Source: CAD feature listing. Evaluate the final solid. Frame: model axes, mm. Face numbers are marked on the shaded views. A direction names the side the tool comes from. Round coordinates to 2 decimals unless told otherwise and drop trailing zeros. Order: outer loops, then holes, each group sorted by start corner. A loop starts at its lowest first (then second) coordinate and runs counter-clockwise, first axis right, second up. Notation, with made-up numbers: (56, 32.5) - (97, 32.5) arc R23 cw to (97, 54.5) - close; hole circle Ø9 at (36, 33). An arc over 180 degrees is marked (long way). Return JSON: item names as keys, results as strings. Group by question number.
1) Mould query, pull axis X, two halves, no side actions, for the marked faces 4, 5 and 6. Classes: pulls with the +X half, pulls with the -X half, needs draft (parallel to the pull), parting line crosses it, or undercut.
2) Section D-D, the plane y = -17.5. Return loops of the section in (x, z).
3) Section B-B, the plane y = -5.5. Return loops of the section in (x, z).
4) Ray query, line 1 (Y direction, x = 7.25, z = 7); line 2 (X direction, y = 0, z = 9.75); line 3 (Z direction, x = -16, y = -18). Return the intervals inside material, ascending. Write a range as from..to.
5) Access query for the marked faces 1, 2 and 3. Directions: +Z, -Z, +X, -X, +Y, -Y. A direction counts if a zero-diameter tool reaches every point of the face in a straight line with its end or side. Return the directions, or none.
6) Section A-A, the plane x = -16. Return loops of the section in (y, z), plus the area to 3 significant figures.
7) Contact query for flat-ended pins moving along their axis: P1, Ø5, axis at x = 16, z = 7, coming from the +Y side; P2, Ø2.5, axis at y = 11.5, z = 5.5, coming from the -X side; P3, Ø2.5, axis at y = 9.5, z = 7.5, coming from the +X side; P4, Ø3.5, axis at x = 14.5, z = 8, coming from the +Y side. Output: stop coordinate, or through.
8) Section C-C, the plane z = 2. Return loops of the section in (x, y).
```python
from build123d import *

# Parameters (mm, degrees)
BOSS_EXTRUDE1_DEPTH         = 14
TAP_DRILL_FOR_M4X0_7_TAP2_D = 3.3
F_12_0_12_DIAMETER_HOLE1_D  = 12
TAP_DRILL_FOR_M5X0_8_TAP1_D = 5.5


with BuildPart() as part:
    # Sketch2 → Boss-Extrude1 (new body)
    with BuildSketch(Plane.XY):
        Polygon((-1, 0), (-1, 14.5), (-9, 14.5), (-9, -17), (-21, -17), (-21, -23), (0, -23), (0, 0), align=None)
    boss_extrude1 = extrude(amount=BOSS_EXTRUDE1_DEPTH)

    # Mirror1: Boss-Extrude1 across plane
    add(boss_extrude1.mirror(Plane(origin=(0, -23, 14), x_dir=(0, 0, 1), z_dir=(-1, 0, 0))))

    # Tap Drill for M4x0.7 Tap2 (through all)
    with Locations(Plane.ZY.offset(9)):
        with Locations((7, 10)):
            Hole(TAP_DRILL_FOR_M4X0_7_TAP2_D / 2)

    # Ø12.0 (12) Diameter Hole1 (through all)
    with Locations(Plane(origin=(0, 0, 0), x_dir=(1, 0, 0), z_dir=(0, 0, -1))):
        with Locations((0, 0)):
            Hole(F_12_0_12_DIAMETER_HOLE1_D / 2)

    # Tap Drill for M5x0.8 Tap1 (through all)
    with Locations(Plane(origin=(0, -23, 0), x_dir=(-1, 0, 0), z_dir=(0, -1, 0))):
        with Locations((-16, -7), (16, -7)):
            Hole(TAP_DRILL_FOR_M5X0_8_TAP1_D / 2)


solid = part.part
```
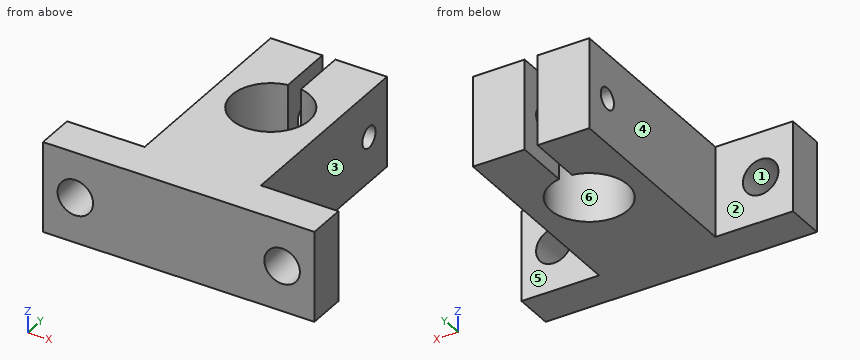
Geometry check:
{
 "1": {"face 4": "pulls with the -X half", "face 5": "needs draft", "face 6": "undercut"},
 "2": {"outline": "(-21, 0) - (21, 0) - (21, 14) - (-21, 14) - close; hole circle Ø5.5 at (-16, 7); hole circle Ø5.5 at (16, 7)"},
 "3": {"outline": "(-9, 0) - (-2.4, 0) - (-2.4, 14) - (-9, 14) - close; (2.4, 0) - (9, 0) - (9, 14) - (2.4, 14) - close"},
 "4": {"line 1": "-23..8.35, 11.65..14.5", "line 2": "-9..-6, 6..9", "line 3": "0..4.25, 9.75..14"},
 "5": {"face 1": "+Y, -Y", "face 2": "+Z, -Z, -X, +Y", "face 3": "+Z, -Z, +X, +Y"},
 "6": {"outline": "(-23, 0) - (-17, 0) - (-17, 4.25) - (-23, 4.25) - close; (-23, 9.75) - (-17, 9.75) - (-17, 14) - (-23, 14) - close", "area": "51.0 mm2"},
 "7": {"P1": "through", "P2": "x = -9", "P3": "x = 9", "P4": "y = -17"},
 "8": {"outline": "(-21, -23) - (21, -23) - (21, -17) - (9, -17) - (9, 14.5) - (1, 14.5) - (1, 5.92) arc R6 cw (long way) to (-1, 5.92) - (-1, 14.5) - (-9, 14.5) - (-9, -17) - (-21, -17) - close"}
}
